```python
from build123d import *

# Parameters (mm, degrees)
F1_DEPTH  = 9
F2_W      = 39
F2_H      = 83
F3_DEPTH  = 5
F6_DEPTH  = 18
F7_W      = 18
F7_H      = 18
F8_DEPTH  = 18
F10_DEPTH = 3
F12_DEPTH = 5
F13_R     = 2.9
F14_DEPTH = 15
F15_W     = 3
F15_H     = 13
F16_DEPTH = 21
F17_DEPTH = 5
F18_W     = 39
F18_H     = 21
F19_DEPTH = 20
F21_DEPTH = 3
F22_R     = 5
F24_DEPTH = 25
F26_R     = 3.6982006044
F26_R_2   = 2.7022216625
F26_R_3   = 3.2521132856
F26_R_4   = 2.4365005618
F27_DEPTH = 3
F29_DEPTH = 25
F30_DEPTH = 2


# Not quite as in the source:
# - a pattern or mirror of a feature is missing from the dataset's text; its kind, count and spacing are read off the source's solid


with BuildPart() as f1:
    # F0 (on Top) → F1 (new body, symmetric)
    with BuildSketch(Plane.XY):
        Polygon((0, 0), (0, 83), (-3, 83), (-3, 3), (-39, 3), (-39, 0), align=None)
    extrude(amount=F1_DEPTH, both=True)

    # F2 (on face) → F3 (join)
    with BuildSketch(Plane.XY.offset(9)):
        with Locations((-19.5, 41.5)):
            Rectangle(F2_W, F2_H)
    extrude(amount=-F3_DEPTH)

    # F5 (on face) → F6 (join)
    with BuildSketch(Plane(origin=(0, 83, 0), x_dir=(-1, 0, 0), z_dir=(0, 1, 0))):
        Polygon((18, 9), (0, 9), (0, -9), (3, -9), (3, 4), (18, 4), align=None)
    extrude(amount=-F6_DEPTH)

    # F7 (on face) → F8 (join)
    with BuildSketch(Plane(origin=(0, 0, -9), x_dir=(1, 0, 0), z_dir=(0, 0, -1))):
        with Locations((-9, -9)):
            Rectangle(F7_W, F7_H)
    f8 = extrude(amount=-F8_DEPTH)

    # F8_copies: F8 across plane
    add(f8.mirror(Plane.ZX.offset(41.5)))

    # F9 (on face) → F10 (join)
    with BuildSketch(Plane(origin=(0, 0, -9), x_dir=(1, 0, 0), z_dir=(0, 0, -1))):
        Polygon((-22, -83), (0, -83), (0, 0), (-39, 0), (-39, -83), align=None)
    extrude(amount=F10_DEPTH)

    # F11 (on face) → F12 (cut, through all)
    with BuildSketch(Plane.XY.offset(9)):
        with BuildLine():
            Line((0, 38.0723795157), (0, 47.9276204843))
            ThreePointArc((0, 47.9276204843), (-28.8418814049, 43), (0, 38.0723795157))
        make_face()
    extrude(amount=-F12_DEPTH, mode=Mode.SUBTRACT)

    # F13 (on face) → F14 (cut)
    with BuildSketch(Plane.YZ):
        with BuildLine():
            Line((10.5, -1.5), (7.6, -1.5))
            ThreePointArc((7.6, -1.5), (8.4493903346, -3.5506096654), (10.5, -4.4))
            Line((10.5, -4.4), (10.5, -1.5))
        make_face()
        with BuildLine():
            ThreePointArc((13.4, -1.5), (10.5, 1.4), (7.6, -1.5))
            Line((7.6, -1.5), (10.5, -1.5))
            Line((10.5, -1.5), (10.5, -4.4))
            ThreePointArc((10.5, -4.4), (12.5506096654, -3.5506096654), (13.4, -1.5))
        make_face()
        Polygon((30, -2.5), (36.5, -9), (36.5, 4), align=None)
        Polygon((36.5, 4), (36.5, -9), (49.5, -9), (49.5, 4), (47.9276204843, 4), (38.0723795157, 4), align=None)
        Polygon((49.5, 4), (49.5, -9), (56, -2.5), align=None)
        with Locations((72.5, -1.5)):
            Circle(F13_R)
    extrude(amount=-F14_DEPTH, mode=Mode.SUBTRACT)

    # F15 (on face) → F16 (join, through all)
    with BuildSketch(Plane(origin=(-18, 0, 0), x_dir=(0, -1, 0), z_dir=(-1, 0, 0))):
        with Locations((-81.5, -2.5)):
            Rectangle(F15_W, F15_H)
    extrude(amount=F16_DEPTH)

    # F4 (on face) → F17 (cut, through all)
    with BuildSketch(Plane.XY.offset(9)):
        with BuildLine():
            ThreePointArc((-22, 62.4), (-23.3435028843, 59.1564971157), (-20.1, 60.5))
            ThreePointArc((-20.1, 60.5), (-20.6564971157, 61.8435028843), (-22, 62.4))
        make_face()
        with BuildLine():
            ThreePointArc((-22, 23.6), (-20.6564971157, 24.1564971157), (-20.1, 25.5))
            ThreePointArc((-20.1, 25.5), (-23.3435028843, 26.8435028843), (-22, 23.6))
        make_face()
    extrude(amount=-F17_DEPTH, mode=Mode.SUBTRACT)

    # F18 (on face) → F19 (join)
    with BuildSketch(Plane.XZ):
        with Locations((-19.5, -1.5)):
            Rectangle(F18_W, F18_H)
    extrude(amount=F19_DEPTH)

    # F20 (on face) → F21 (join)
    with BuildSketch(Plane.XZ.offset(20)):
        Polygon((0, 30), (-39, 30), (-39, 9), (-39, -12), (-39, -33), (0, -33), (0, -12), (0, 9), align=None)
    extrude(amount=F21_DEPTH)

    # F22
    f22_edges = [f1.edges().sort_by_distance(p)[0] for p in [
        (-19.5, -20, -12),
        (-19.5, -20, 9),
    ]]
    fillet(f22_edges, radius=F22_R)

    # F23 (on face) → F24 (cut)
    with BuildSketch(Plane.XZ.offset(23)):
        with BuildLine():
            Line((-32, 21.1), (-32, 23))
            Line((-32, 23), (-30.1, 23))
            ThreePointArc((-30.1, 23), (-33.3435028843, 24.3435028843), (-32, 21.1))
        make_face()
        with BuildLine():
            Line((-30.1, 23), (-32, 23))
            Line((-32, 23), (-32, 21.1))
            ThreePointArc((-32, 21.1), (-30.6564971157, 21.6564971157), (-30.1, 23))
        make_face()
        with BuildLine():
            ThreePointArc((-5.1, 23), (-7, 24.9), (-8.9, 23))
            Line((-8.9, 23), (-7, 23))
            Line((-7, 23), (-7, 21.1))
            ThreePointArc((-7, 21.1), (-5.6564971157, 21.6564971157), (-5.1, 23))
        make_face()
        with BuildLine():
            Line((-7, 23), (-8.9, 23))
            ThreePointArc((-8.9, 23), (-8.3435028843, 21.6564971157), (-7, 21.1))
            Line((-7, 21.1), (-7, 23))
        make_face()
        with BuildLine():
            Line((-32, -26), (-32, -24.1))
            ThreePointArc((-32, -24.1), (-33.3435028843, -27.3435028843), (-30.1, -26))
            Line((-30.1, -26), (-32, -26))
        make_face()
        with BuildLine():
            ThreePointArc((-30.1, -26), (-30.6564971157, -24.6564971157), (-32, -24.1))
            Line((-32, -24.1), (-32, -26))
            Line((-32, -26), (-30.1, -26))
        make_face()
        with BuildLine():
            ThreePointArc((-5.1, -26), (-5.6564971157, -24.6564971157), (-7, -24.1))
            Line((-7, -24.1), (-7, -26))
            Line((-7, -26), (-8.9, -26))
            ThreePointArc((-8.9, -26), (-7, -27.9), (-5.1, -26))
        make_face()
        with BuildLine():
            Line((-7, -26), (-7, -24.1))
            ThreePointArc((-7, -24.1), (-8.3435028843, -24.6564971157), (-8.9, -26))
            Line((-8.9, -26), (-7, -26))
        make_face()
    extrude(amount=-F24_DEPTH, mode=Mode.SUBTRACT)

    # F26 (on face) → F27 (join, through all)
    with BuildSketch(Plane(origin=(0, -20, 0), x_dir=(-1, 0, 0), z_dir=(0, 1, 0))):
        with Locations((32, 23)):
            Circle(F26_R)
        with Locations((7, 23)):
            Circle(F26_R_2)
        with Locations((31.5193422139, -25.7969032973)):
            Circle(F26_R_3)
        with Locations((7.0765195414, -26.2656044215)):
            Circle(F26_R_4)
    extrude(amount=-F27_DEPTH)

    # F28 (on face) → F29 (cut)
    with BuildSketch(Plane(origin=(0, -20, 0), x_dir=(-1, 0, 0), z_dir=(0, 1, 0))):
        with BuildLine():
            ThreePointArc((19.5, 15.6), (20.8435028843, 16.1564971157), (21.4, 17.5))
            ThreePointArc((21.4, 17.5), (20.8435028843, 18.8435028843), (19.5, 19.4))
            Line((19.5, 19.4), (19.5, 17.5))
            Line((19.5, 17.5), (19.5, 15.6))
        make_face()
        with BuildLine():
            ThreePointArc((21.4, -20.5), (20.8435028843, -19.1564971157), (19.5, -18.6))
            Line((19.5, -18.6), (19.5, -20.5))
            Line((19.5, -20.5), (19.5, -22.4))
            ThreePointArc((19.5, -22.4), (20.8435028843, -21.8435028843), (21.4, -20.5))
        make_face()
        with BuildLine():
            Line((19.5, -20.5), (19.5, -18.6))
            ThreePointArc((19.5, -18.6), (17.6, -20.5), (19.5, -22.4))
            Line((19.5, -22.4), (19.5, -20.5))
        make_face()
        with BuildLine():
            Line((19.5, 17.5), (19.5, 19.4))
            ThreePointArc((19.5, 19.4), (17.6, 17.5), (19.5, 15.6))
            Line((19.5, 15.6), (19.5, 17.5))
        make_face()
    extrude(amount=-F29_DEPTH, mode=Mode.SUBTRACT)

    # F30 (add): a face of the model
    f30_faces = [f1.faces().sort_by_distance(p)[0] for p in [
        (-19.5, -23, -1.5),
    ]]
    extrude(f30_faces, amount=F30_DEPTH)


solid = f1.part
```
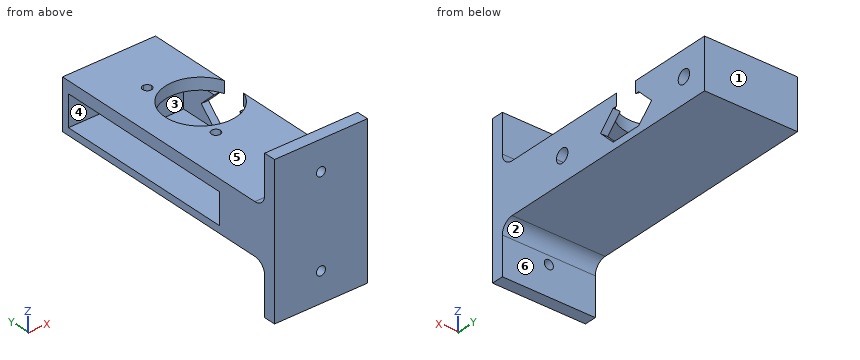
Geometry check sheet. Reference: the model listing, model coordinates, mm. Face numbers are marked on the shaded views. A direction names the side the tool comes from. Give positions to 0.01 mm unless a question says otherwise; leave off trailing zeros. Order: outer loops, then holes, each group sorted by start corner. A loop starts at its lowest first (then second) coordinate and runs counter-clockwise, first axis right, second up. Notation, with made-up numbers: (0, 19) -> (55, 19) arc R9 ccw to (55, 26) -> close; hole circle Ø1 at (50.25, 80.5). An arc over 180 degrees is marked (long way). Write each question's results on one line, items separated by ' | '. Start each with the question number.
(1) Sectioned sample at A-A (y = 43). Enter the section's corners in (x, z), plus the area to 3 significant figures.
(2) Scan lines: line 1 (Z direction, x = -19.5, y = -23.8); line 2 (Y direction, x = -14, z = 5.9); line 3 (Z direction, x = -27.5, y = 18). Record each from-to range of solid material in increasing order.
(3) Mould release check, pull along Z, two halves, no side actions. Record for the marked faces 1, 2 and 3: pulls with the +Z half, pulls with the -Z half, needs draft (parallel to the pull), parting line crosses it, or undercut.
(4) Sectioned sample at C-C (x = -7.5). Enter the section's corners in (y, z), plus the area to 3 significant figures.
(5) Sectioned sample at D-D (y = 22.5). Enter the section's corners in (x, z).
(6) Sectioned sample at B-B (z = 17.5). Enter the section's corners in (x, y).
(7) Gauge pin test, flat ends, axial feed: P1, Ø3, axis at x = -32.5, y = 17, coming from the +Z side; P2, Ø6, axis at x = -22.5, y = 48, coming from the +Z side; P3, Ø10.5, axis at y = 28, z = -1.5, coming from the -X side; P4, Ø3, axis at x = -19.5, z = -20.5, coming from the -Y side. Record the tip position at first contact, or that the pin passes through.
(8) Access from +Z, -Z, +X, -X, +Y, -Y to the whole of each face (thin tool, end or side, straight path). Record for the marked faces 4, 5 and 6.
Answer below:
1) outline: (-39, -12) -> (0, -12) -> (0, -9) -> (-39, -9) -> close; (-39, 4) -> (-28.84, 4) -> (-28.84, 9) -> (-39, 9) -> close | area: 168 mm2
2) line 1: -33 to -22.4, -18.6 to 15.6, 19.4 to 30 | line 2: -25 to 28.16, 57.84 to 83 | line 3: -12 to -9, 4 to 9
3) face 1: needs draft | face 2: pulls with the -Z half | face 3: undercut
4) outline: (-25, -33) -> (-20, -33) -> (-20, -17) arc R5 cw to (-15, -12) -> (83, -12) -> (83, 9) -> (56.34, 9) -> (56.34, 4) -> (65, 4) -> (65, -9) -> (18, -9) -> (18, 4) -> (29.66, 4) -> (29.66, 9) -> (-15, 9) arc R5 cw to (-20, 14) -> (-20, 30) -> (-25, 30) -> close; hole circle Ø5.8 at (10.5, -1.5); hole circle Ø5.8 at (72.5, -1.5) | area: 1,690 mm2
5) outline: (-39, -12) -> (0, -12) -> (0, 9) -> (-39, 9) -> (-39, 4) -> (-3, 4) -> (-3, -9) -> (-39, -9) -> close
6) outline: (-39, -25) -> (-21.4, -25) -> (-21.4, -20) -> (-39, -20) -> close; (-17.6, -25) -> (0, -25) -> (0, -20) -> (-17.6, -20) -> close
7) P1: z = 9 | P2: z = -9 | P3: x = -3 | P4: through
8) face 4: -X | face 5: +Z, +X, -X, +Y | face 6: -Z, +X, -X, +Y
